The model under review builds one solid part; all positions refer to its coordinate system, in mm. A direction names the side the tool comes from. Round coordinates to 2 decimals unless told otherwise and drop trailing zeros. Write each loop counter-clockwise with the first axis right and the second up, starting at its lowest first coordinate (ties: lowest second). Pieces come first, ordered by that corner, then holes. Notation, with made-up numbers: (21.5, 19.5) -> (34.5, 19.5) arc R33 cw to (34.5, 48.5) -> close; hole circle Ø4 at (9, 82). An arc over 180 degrees is marked (long way). Return JSON: item names as keys, results as strings. Group by question number.
1. Take a section at A-A, the plane z = 0. Write out the cut boundary in (x, y).
2. Mouldability with a two-part tool opening along X and no side actions: class faces 4 (the flat face through (2, 11, 0)), 5 (the flat face through (-16, 53, 0)), 6 (the flat face through (12, 79, 13)), 7 (the flat face through (0, 9, 0)) as pulls with the +X half, pulls with the -X half, needs draft (parallel to the pull), parting line crosses it, or undercut.
3. Take a section at B-B, the plane y = 79. Write out the cut boundary in (x, z).
4. Take a section at D-D, the plane x = 13.5. Write out the cut boundary in (y, z).
5. For line 1 along Z through (x, y) = (-10.5, 79); line 2 along Y through (x, z) = (-12, 0); line 3 along X through (y, z) = (15.5, -18), list the stretches that pass through material, from the lowest coordinate up. Write a range as from..to.
6. Tool access review of faces 1 (the flat face through (16, 53, 0)), 2 (the cylindrical face through (-10.787, 3.451, 2.395)), 3 (the flat face through (-12, 79, 17)): name each direction out of +Z, -Z, +X, -X, +Y, -Y from which nothing blocks a thin tool from reaching the whole face with its end or side.
7. Clearance check with flat-ended pins moving along their axes: P1, Ø13.5, axis at x = 0, z = 0, coming from the -Y side; P2, Ø4.5, axis at x = 1, z = 7, coming from the +Y side; P3, Ø12, axis at y = 54, z = -2, coming from the -X side; P4, Ø13.5, axis at y = 79, z = 0, coming from the -X side. State where each tip first meets the part, or that it passes through.
8. Take a section at C-C, the plane y = 54. Write out the cut boundary in (x, z), then the cut area to 3 significant figures.
from build123d import *

# Parameters (mm, degrees)
SKETCH1_R               = 30
BOSS_EXTRUDE1_DEPTH     = 14
SKETCH2_R               = 11.05
CUT_EXTRUDE1_DEPTH      = 7
SKETCH5_W               = 7.5
SKETCH5_H               = 40
BOSS_EXTRUDE2_DEPTH     = 80
FILLET1_R               = 10
CUT_EXTRUDE3_DEPTH      = 109.866891202
CUT_EXTRUDE3_DEPTH_BACK = 109.866891202
SKETCH7_R               = 11.05
CUT_EXTRUDE4_START      = -5
CUT_EXTRUDE4_DEPTH      = 5
CUT_EXTRUDE5_REACH      = 110.867
SKETCH9_W               = 4
SKETCH9_H               = 5


with BuildPart() as part:
    # Sketch1 → Boss-Extrude1 (new body)
    with BuildSketch(Plane(origin=(0, 0, 0), x_dir=(1, 0, 0), z_dir=(0, 1, 0))):
        with Locations(Location((0, 0, 0), (0, 0, 90))):
            Circle(SKETCH1_R)
    extrude(amount=BOSS_EXTRUDE1_DEPTH)

    # Sketch2 → Cut-Extrude1 (cut)
    with BuildSketch(Plane.XZ):
        with Locations(Location((0, 0, 0), (0, 0, 270))):
            Circle(SKETCH2_R)
    extrude(amount=-CUT_EXTRUDE1_DEPTH, mode=Mode.SUBTRACT)

    # Sketch5 → Boss-Extrude2 (add)
    with BuildSketch(Plane(origin=(0, 14, 0), x_dir=(1, 0, 0), z_dir=(0, 1, 0))):
        with Locations((-12.25, 0)):
            Rectangle(SKETCH5_W, SKETCH5_H)
        with Locations((12.25, 0)):
            Rectangle(SKETCH5_W, SKETCH5_H)
    extrude(amount=BOSS_EXTRUDE2_DEPTH)

    # Fillet1
    fillet1_edges = [part.edges().sort_by_distance(p)[0] for p in [
        (-12.25, 94, 20),
        (-12.25, 94, -20),
        (12.25, 94, 20),
        (12.25, 94, -20),
    ]]
    fillet(fillet1_edges, radius=FILLET1_R)

    # Sketch7 → Cut-Extrude3 (cut, two sides: drawn at the far end of the back side and taken through both)
    with BuildSketch(Plane.ZY.offset(16).offset(-CUT_EXTRUDE3_DEPTH_BACK)):
        with Locations((0, 79)):
            Circle(SKETCH7_R)
    extrude(amount=CUT_EXTRUDE3_DEPTH + CUT_EXTRUDE3_DEPTH_BACK, mode=Mode.SUBTRACT)

    # Sketch8 → Cut-Extrude4 (cut)
    with BuildSketch(Plane(origin=(0, 14, 0), x_dir=(1, 0, 0), z_dir=(0, 1, 0)).offset(CUT_EXTRUDE4_START)):
        with BuildLine():
            Line((2, 29.933259094), (2, -29.933259094))
            ThreePointArc((2, -29.933259094), (0, -30), (-2, -29.933259094))
            Line((-2, -29.933259094), (-2, 29.933259094))
            ThreePointArc((-2, 29.933259094), (0, 30), (2, 29.933259094))
        make_face()
    extrude(amount=CUT_EXTRUDE4_DEPTH, mode=Mode.SUBTRACT)

    # Cut-Extrude5: up to this face of the body (flat: up to its plane)
    cut_extrude5_end = Plane(part.part.faces().sort_by_distance((16, 49.957843981, 0))[0])
    # Sketch9 → Cut-Extrude5 (cut, up to the picked face)
    with BuildSketch(Plane.ZY.offset(16), mode=Mode.PRIVATE) as cut_extrude5_sk1:
        with Locations((15, 79)):
            Rectangle(SKETCH9_W, SKETCH9_H)
    cut_extrude5_tool1 = split(extrude(cut_extrude5_sk1.sketch, amount=-CUT_EXTRUDE5_REACH, mode=Mode.PRIVATE), bisect_by=cut_extrude5_end, keep=Keep.BOTH, mode=Mode.PRIVATE)
    add(cut_extrude5_tool1.solids().sort_by(Axis((-16, 79, 15), (1, 0, 0)))[0], mode=Mode.SUBTRACT)


solid = part.part
Output:
{
 "1": {"outline": "(-30, 0) -> (-11.05, 0) -> (-11.05, 7) -> (11.05, 7) -> (11.05, 0) -> (30, 0) -> (30, 14) -> (16, 14) -> (16, 67.95) -> (8.5, 67.95) -> (8.5, 14) -> (2, 14) -> (2, 9) -> (-2, 9) -> (-2, 14) -> (-8.5, 14) -> (-8.5, 67.95) -> (-16, 67.95) -> (-16, 14) -> (-30, 14) -> close; (-16, 90.05) -> (-8.5, 90.05) -> (-8.5, 94) -> (-16, 94) -> close; (8.5, 90.05) -> (16, 90.05) -> (16, 94) -> (8.5, 94) -> close"},
 "2": {"face 4": "undercut", "face 5": "pulls with the -X half", "face 6": "needs draft", "face 7": "undercut"},
 "3": {"outline": "(-16, -20) -> (-8.5, -20) -> (-8.5, -11.05) -> (-16, -11.05) -> close; (-16, 11.05) -> (-8.5, 11.05) -> (-8.5, 13) -> (-16, 13) -> close; (-16, 17) -> (-8.5, 17) -> (-8.5, 20) -> (-16, 20) -> close; (8.5, -20) -> (16, -20) -> (16, -11.05) -> (8.5, -11.05) -> close; (8.5, 11.05) -> (16, 11.05) -> (16, 13) -> (8.5, 13) -> close; (8.5, 17) -> (16, 17) -> (16, 20) -> (8.5, 20) -> close"},
 "4": {"outline": "(0, -26.79) -> (14, -26.79) -> (14, -20) -> (84, -20) arc R10 ccw to (94, -10) -> (94, 10) arc R10 ccw to (84, 20) -> (14, 20) -> (14, 26.79) -> (0, 26.79) -> close; hole circle Ø22.1 at (79, 0); hole (76.5, 13) -> (81.5, 13) -> (81.5, 17) -> (76.5, 17) -> close"},
 "5": {"line 1": "z = -20..-11.05, 11.05..13, 17..20", "line 2": "y = 0..67.95, 90.05..94", "line 3": "x = -16..-8.5, 8.5..16"},
 "6": {"face 1": "+Z, -Z, +X, +Y", "face 2": "-Y", "face 3": "+X, -X"},
 "7": {"P1": "stops at y = 7", "P2": "stops at y = 14", "P3": "stops at x = -16", "P4": "passes through"},
 "8": {"outline": "(-16, -20) -> (-8.5, -20) -> (-8.5, 20) -> (-16, 20) -> close; (8.5, -20) -> (16, -20) -> (16, 20) -> (8.5, 20) -> close", "area": "600 mm^2"}
}
